from build123d import *

# Parameters (mm, degrees)
F0_W     = 254
F0_H     = 101.6
F0_R     = 4.7625
F1_DEPTH = 25.4
F2_R     = 33.02
F2_R_2   = 4.7625
F2_R_3   = 25.4
F3_DEPTH = 19.05
F4_W     = 106.8471033573
F4_H     = 12.1652636021
F5_DEPTH = 101.601
F6_R     = 2.54


with BuildPart() as f1:
    # F0 (on Top) → F1 (new body)
    with BuildSketch(Plane.XY):
        Rectangle(F0_W, F0_H)
        with Locations((-76.2, 0)):
            Circle(F0_R, mode=Mode.SUBTRACT)
        with Locations((76.2, 0)):
            Circle(F0_R, mode=Mode.SUBTRACT)
    extrude(amount=F1_DEPTH)

    # F2 (on face) → F3 (cut)
    with BuildSketch(Plane.XY.offset(25.4)):
        with Locations((-76.2, 0)):
            Circle(F2_R)
        with Locations((-76.2, 0)):
            Circle(F2_R_2, mode=Mode.SUBTRACT)
        with Locations((76.2, 0)):
            Circle(F2_R_3)
        with Locations((76.2, 0)):
            Circle(F2_R_2, mode=Mode.SUBTRACT)
    extrude(amount=-F3_DEPTH, mode=Mode.SUBTRACT)

    # F4 (on face) → F5 (cut, through all)
    with BuildSketch(Plane.XZ.offset(50.8)):
        Polygon((-138.9647424221, 56.2476329505), (-157.312899828, 13.2347363979), (-127, 13.2347363979), (-127, 25.4), (-20.1528966427, 25.4), (-20.1528966427, 66.1736875772), align=None)
        with Locations((-73.5764483213, 19.3173681989)):
            Rectangle(F4_W, F4_H)
    extrude(amount=-F5_DEPTH, mode=Mode.SUBTRACT)

    # F6
    f6_edges = [f1.edges().sort_by_distance(p)[0] for p in [
        (-73.576448, -50.8, 13.234736),
        (53.423552, -50.8, 25.4),
        (-20.152897, -50.8, 19.317368),
        (127, -50.8, 12.7),
        (0, -50.8, 0),
        (127, 0, 25.4),
        (127, 50.8, 12.7),
        (127, 0, 0),
        (53.423552, 50.8, 25.4),
        (-20.152897, 0, 25.4),
        (50.8, 0, 25.4),
        (-109.22, 0, 13.234736),
        (-20.152897, 50.8, 19.317368),
        (-73.576448, 50.8, 13.234736),
        (0, 50.8, 0),
        (-127, 0, 0),
        (-127, -50.8, 6.617368),
        (-127, 0, 13.234736),
        (-127, 50.8, 6.617368),
        (-20.152897, 0, 13.234736),
    ]]
    fillet(f6_edges, radius=F6_R)


solid = f1.part
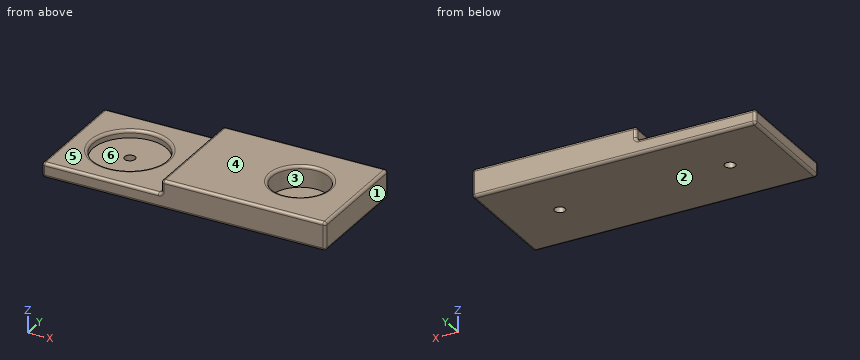
Design review of the part built by this model. Coordinates are the model's own, in mm. Face numbers are marked on the shaded views. A direction names the side the tool comes from. Round coordinates to 2 decimals unless told otherwise and drop trailing zeros. Loops run counter-clockwise (first coordinate to the right, second up) from the corner with the lowest first, then second, coordinate; pieces in that order, holes last. Notation, with made-up numbers: (-14.75, 73) - (-5.75, 73) arc R32 ccw to (-5.75, 103) - close; hole circle Ø10 at (3.25, 59.25). An arc over 180 degrees is marked (long way). One line per item, written item: value. Start each with the question number.
1) Insertion check: pin 1 Ø5.5 at (y, z) = (-12, 18.5) entering from -X; pin 2 Ø3 at (x, y) = (-99.5, 8.5) entering from +Z; pin 3 Ø11 at (x, y) = (-76.2, 0) entering from -Z; pin 4 Ø4 at (y, z) = (33, 14.5) entering from -X. Each pin has a flat end and moves straight along its axis. Give the tip position at first contact, or say it passes through.
2) Consider section C-C on x = 76.2. Give the boundary of the cut face in (y, z).
3) Consider section D-D on y = 41. Give the boundary of the cut face in (x, z).
4) Consider section B-B on z = 19.5. Give the boundary of the cut face in (x, y).
5) For the marked faces 4, 5 and 6, list the 3-axis set-ups (+Z, -Z, +X, -X, +Y, -Y) from which the entire face can be reached by the end or side of a thin tool; tool diameter is ignored.
6) To check wall thickness, follow L1, parallel to Y at x = -76.2, z = 3.75; L2, parallel to Y at x = 76.2, z = 13; L3, parallel to X at y = 15.5, z = 8.5. State the ranges of each line that lie inside material, in increasing order. Write a range as from..to.
7) Draft analysis for pull direction X (two halves, no side actions). For the marked faces 1, 2 and 3, state which applies: +X half, -X half, draft (parallel to the pull), parting line (faces both ways), or undercut.
8) Consider section A-A on y = 0. Give the number of separate pieces and of enclosed holes in the cut face, then the cut area to 3 significant figures.
Reported:
1. pin 1: stops at x = -20.15
1. pin 2: stops at z = 6.35
1. pin 3: stops at z = 0
1. pin 4: stops at x = -126.25
2. outline: (-50.8, 2.54) arc R2.54 ccw to (-48.26, 0) - (-4.76, 0) - (-4.76, 6.35) - (-25.4, 6.35) - (-25.4, 22.86) arc R2.54 ccw to (-27.94, 25.4) - (-48.26, 25.4) arc R2.54 ccw to (-50.8, 22.86) - close; (4.76, 0) - (48.26, 0) arc R2.54 ccw to (50.8, 2.54) - (50.8, 22.86) arc R2.54 ccw to (48.26, 25.4) - (27.94, 25.4) arc R2.54 ccw to (25.4, 22.86) - (25.4, 6.35) - (4.76, 6.35) - close
3. outline: (-127, 2.54) arc R2.54 ccw to (-124.46, 0) - (124.46, 0) arc R2.54 ccw to (127, 2.54) - (127, 22.86) arc R2.54 ccw to (124.46, 25.4) - (-17.61, 25.4) arc R2.54 ccw to (-20.15, 22.86) - (-20.15, 15.77) arc R2.54 cw to (-22.69, 13.23) - (-124.46, 13.23) arc R2.54 ccw to (-127, 10.69) - close
4. outline: (-20.15, -48.26) arc R2.54 ccw to (-17.61, -50.8) - (124.46, -50.8) arc R2.54 ccw to (127, -48.26) - (127, 48.26) arc R2.54 ccw to (124.46, 50.8) - (-17.61, 50.8) arc R2.54 ccw to (-20.15, 48.26) - close; hole circle Ø50.8 at (76.2, 0)
5. face 4: +Z, +X, -X, +Y, -Y
5. face 5: +Z, -X, +Y, -Y
5. face 6: +Z
6. L1: y = -50.8..-4.76, 4.76..50.8
6. L2: y = -50.8..-25.4, 25.4..50.8
6. L3: x = -127..-105.36, -47.04..56.08, 96.32..127
7. face 1: +X half
7. face 2: draft
7. face 3: undercut
8. separate pieces: 3
8. enclosed holes: 0
8. area: 3,600 mm^2
